from build123d import *

# Parameters (mm, degrees)
F1_DEPTH = 35
F2_F1_R  = 10
F2_F2_R  = 10


with BuildPart() as f1:
    # F0 (on Front) → F1 (new body)
    with BuildSketch(Plane.XZ):
        with BuildLine():
            ThreePointArc((-0.0047558207, 48.9411353783), (-31.5398699376, 57.380504031), (-39.9857325354, 25.8471285283))
            Line((-39.9857325354, 25.8471285283), (0.0142674646, -43.4349037745))
            Line((0.0142674646, -43.4349037745), (40.0142674646, 25.8471285283))
            ThreePointArc((40.0142674646, 25.8471285283), (31.5541374022, 57.4077646413), (-0.0047558207, 48.9411353783))
        make_face()
        with BuildLine():
            ThreePointArc((-3.643705829, 6.997927092), (-3.7871096163, 19.9786310917), (7.4790206276, 13.5293249041))
            ThreePointArc((7.4790206276, 13.5293249041), (6.4493061876, 9.7422152878), (3.643705829, 6.997927092))
            Line((3.643705829, 6.997927092), (4.1987560689, 6.997927092))
            Line((4.1987560689, 6.997927092), (4.1987560689, -6.997927092))
            Line((4.1987560689, -6.997927092), (-4.1987560689, -6.997927092))
            Line((-4.1987560689, -6.997927092), (-4.1987560689, 6.997927092))
            Line((-4.1987560689, 6.997927092), (-3.643705829, 6.997927092))
        make_face(mode=Mode.SUBTRACT)
        with BuildLine():
            ThreePointArc((0, 25.8471285283), (-3.0951138699, 37.3934950566), (-0.0047558207, 48.9411353783))
            ThreePointArc((-0.0047558207, 48.9411353783), (3.0929066858, 37.3947693749), (0, 25.8471285283))
        make_face(mode=Mode.SUBTRACT)
        with BuildLine():
            ThreePointArc((0, 25.8471285283), (3.0929066858, 37.3947693749), (-0.0047558207, 48.9411353783))
            ThreePointArc((-0.0047558207, 48.9411353783), (-3.0951138699, 37.3934950566), (0, 25.8471285283))
        make_face()
    extrude(amount=F1_DEPTH)

    # F2: fillet of radius 10 on 4 edges, made by hand

    # F2_f1
    f2_f1_edges = [f1.edges().sort_by_distance(p)[0] for p in [
        (-0.0047558207, -17.5, 48.9411353783),
    ]]
    fillet(f2_f1_edges, radius=F2_F1_R)

    # F2_f2
    f2_f2_edges = [f1.edges().sort_by_distance(p)[0] for p in [
        (-35.2672128577, 0, 54.7003379421),
        (-35.2672128577, -35, 54.7003379421),
        (-19.9857325354, -35, -8.7938876231),
        (-19.9857325354, 0, -8.7938876231),
        (-0.0065856085, -35, 53.761031934),
        (-0.0065856085, 0, 53.761031934),
    ]]
    fillet(f2_f2_edges, radius=F2_F2_R)


solid = f1.part
Could you check a few things on this model? Use its own coordinates, in mm. A direction names the side the tool comes from. Round coordinates to 2 decimals unless told otherwise and drop trailing zeros. Put each result on its own line as item: value. Start each with the question number.
(1) I need wall thicknesses on probe 1 along Z at (x, y) = (0, -11); probe 2 along Z at (x, y) = (0, -8.5); probe 3 along X at (y, z) = (-3.5, 16). Which ranges of each line are inside material? Lowest first, please.
(2) For faces 1 (the flat face through (4.199, -17, 0)), 2 (the cylindrical face through (-17.1, -32.15, -7.78)), which set-ups out of +Z, -Z, +X, -X, +Y, -Y let a thin tool reach every point of the face, with its end or its side?
(3) Thinking about a two-plate mould opening in Z: for faces 3 (the flat face through (19.734, -17.395, -9.279)), 4 (the flat face through (0, -35, 22)), 5 (the flat face through (0, -17, -6.998)), which applies, released by +Z, released by -Z, zero draft, split by the parting line, or undercut?
(4) Will these pins go through, and if not, where does the flat tip stop? pin 1 (11 mm diameter, centred on y = -17, z = 3, fed in from +X); pin 2 (8 mm diameter, centred on y = -21.5, z = 46.5, fed in from -X); pin 3 (5 mm diameter, centred on x = 14, y = -3.5, fed in from -Z).
Here are the results:
1. probe 1: z = -43.41 to -7, 21.01 to 53.76
1. probe 2: z = -43.18 to -7, 21.01 to 53.65
1. probe 3: x = -31.53 to -7.06, 7.06 to 31.56
2. face 1: +Y, -Y
2. face 2: -Z, -X, -Y
3. face 3: released by -Z
3. face 4: zero draft
3. face 5: undercut
4. pin 1: stops at x = 30
4. pin 2: stops at x = -42.51
4. pin 3: stops at z = -20
